Design review of the part built by this model. Coordinates are the model's own, in mm. Round coordinates to 2 decimals unless told otherwise and drop trailing zeros. Order: outer loops, then holes, each group sorted by start corner. A loop starts at its lowest first (then second) coordinate and runs counter-clockwise, first axis right, second up. Notation, with made-up numbers: (24, 4) - (56, 4) arc R19 ccw to (56, 39) - close; hole circle Ø8 at (21, -35). An arc over 180 degrees is marked (long way). Use CSV: the item, a comma, the result in double quotes. Start each with the question number.
from build123d import *

# Parameters (mm, degrees)
EXTRUDE_1_DEPTH     = 10
CUT_EXTRUDE_1_DEPTH = 28.77666362
FILLET_1_R          = 0.8
SKETCH_3_R          = 1.7
SKETCH_3_R_2        = 1.9
CUT_EXTRUDE_2_DEPTH = 10


with BuildPart() as part:
    # 草图1 → 凸台-拉伸1 (new body)
    with BuildSketch(Plane(origin=(0, 0, 0), x_dir=(0, 0, -1), z_dir=(1, 0, 0))):
        with BuildLine():
            Line((-10.635898576, 16.411798263), (2.964101424, 16.411798263))
            Line((2.964101424, 16.411798263), (14.164101424, 16.411798263))
            ThreePointArc((14.164101424, 16.411798263), (16.235169236, 11.411798263), (14.164101424, 6.411798263))
            Line((14.164101424, 6.411798263), (2.964101424, 6.411798263))
            Line((2.964101424, 6.411798263), (-10.635898576, 6.411798263))
            Line((-10.635898576, 6.411798263), (-21.835898576, 6.411798263))
            ThreePointArc((-21.835898576, 6.411798263), (-23.906966388, 11.411798263), (-21.835898576, 16.411798263))
            Line((-21.835898576, 16.411798263), (-10.635898576, 16.411798263))
        make_face()
    extrude(amount=EXTRUDE_1_DEPTH)

    # 草图2 → 切除-拉伸1 (cut, through all)
    with BuildSketch(Plane.XZ.offset(-6.411798263)):
        with BuildLine():
            Line((10, 9.782326075), (10, -2.110528923))
            ThreePointArc((10, -2.110528923), (4.8, 3.835898576), (10, 9.782326075))
        make_face()
    extrude(amount=-CUT_EXTRUDE_1_DEPTH, mode=Mode.SUBTRACT)

    # 圆角1
    fillet_1_edges = [part.edges().sort_by_distance(p)[0] for p in [
        (10, 11.411798263, -2.110528923),
        (10, 11.411798263, 9.782326075),
    ]]
    fillet(fillet_1_edges, radius=FILLET_1_R)

    # 草图3 → 切除-拉伸2 (cut)
    with BuildSketch(Plane(origin=(10, 0, 0), x_dir=(0, 0, -1), z_dir=(1, 0, 0))):
        with Locations((-16.835898576, 11.411798263)):
            Circle(SKETCH_3_R)
        with Locations((9.164101424, 11.411798263)):
            Circle(SKETCH_3_R_2)
    extrude(amount=-CUT_EXTRUDE_2_DEPTH, mode=Mode.SUBTRACT)


solid = part.part
Q1. Take a section at C-C (y = 12.25). State the section outline as (x, z) points.
Q2. Take a section at D-D (x = 6). State the section outline as (y, z) points, plus the area to 3 significant figures.
Q3. The part is to be moulded in two halves that separate along Y. For faces 1 (the flat face through (4, 16.412, 4)), 2 (the cylindrical face through (5.07, 13.01, -10.19)), 3 (the flat face through (10, 11, 19)), 4 (the cylindrical face through (5.07, 11.487, 18.534)), say which applies: +Y half, -Y half, draft (parallel to the pull), parting line (faces both ways), or undercut.
Q4. Take a section at B-B (z = -9.5). State the section outline as (x, y) points.
Q5. Clearance check with flat-ended pins moving along their axes: pin 1 (3.5 mm diameter, centred on y = 11.41, z = -9.16, fed in from +X); pin 2 (6 mm diameter, centred on x = 7, y = 15, fed in from +Z); pin 3 (3 mm diameter, centred on x = 8.5, y = 14.5, fed in from +Z). State where each tip first meets the part, or that it passes through.
Q6. For L1, parallel to Z at x = 8.5, y = 11.5; L2, parallel to Z at x = 3.5, y = 11; L3, parallel to Z at x = 8, y = 10.5, list the stretches that pass through material, from the lowest coordinate up. Write a range as [from, to].
Q7. Take a section at A-A (x = 8). State the section outline as (y, z) points.
Findings below:
1,outline,"(0, -16.19) - (10, -16.19) - (10, -10.87) - (0, -10.87) - close; (0, -7.46) - (10, -7.46) - (10, -2.77) arc R0.8 ccw to (9.39, -2) arc R6 cw to (9.39, 9.67) arc R0.8 ccw to (10, 10.44) - (10, 15.36) - (0, 15.36) - close; (0, 18.31) - (10, 18.31) - (10, 23.86) - (0, 23.86) - close"
2,outline,"(6.41, -14.16) arc R7.07 ccw to (16.41, -14.16) - (16.41, 0.24) - (6.41, 0.24) - close; (6.41, 7.44) - (16.41, 7.44) - (16.41, 21.84) arc R7.07 ccw to (6.41, 21.84) - close; hole circle Ø3.8 at (11.41, -9.16); hole circle Ø3.4 at (11.41, 16.84)"
2,area,"296 mm^2"
3,face 1,"+Y half"
3,face 2,"undercut"
3,face 3,"draft"
3,face 4,"undercut"
4,outline,"(0, 6.41) - (10, 6.41) - (10, 9.54) - (0, 9.54) - close; (0, 13.28) - (10, 13.28) - (10, 16.41) - (0, 16.41) - close"
5,pin 1,"passes through"
5,pin 2,"stops at z = 23.88"
5,pin 3,"stops at z = 23.73"
6,L1,"z = [-16.23, -11.06], [-7.27, -1.71], [9.38, 15.14], [18.53, 23.91]"
6,L2,"z = [-16.22, -11.02], [-7.31, 15.19], [18.49, 23.89]"
6,L3,"z = [-16.18, -10.83], [-7.5, -1.47], [9.14, 15.4], [18.27, 23.85]"
7,outline,"(6.41, -14.16) arc R7.07 ccw to (16.41, -14.16) - (16.41, -1.47) - (6.41, -1.47) - close; (6.41, 9.14) - (16.41, 9.14) - (16.41, 21.84) arc R7.07 ccw to (6.41, 21.84) - close; hole circle Ø3.8 at (11.41, -9.16); hole circle Ø3.4 at (11.41, 16.84)"
